Read the model definition and answer for the solid it produces. Units are mm, in the model's axes. Face numbers are marked on the shaded views. A direction names the side the tool comes from. Coordinates: 2 decimals unless noted, no trailing zeros. Order: outer loops, then holes, each group sorted by start corner. A loop starts at its lowest first (then second) coordinate and runs counter-clockwise, first axis right, second up. Notation, with made-up numbers: (29.5, 19.25) -> (77.5, 19.25) arc R30 ccw to (77.5, 45.25) -> close; hole circle Ø4 at (86.5, 56). An arc over 180 degrees is marked (long way). Answer as a JSON object with one key per item and string values. Group by question number.
1) A tool of negligible diameter and unlimited length cuts with its end or side. For the marked faces 1 and 2, from which of +Z, -Z, +X, -X, +Y, -Y can it reach the whole face along a straight path? Write none if from no direction.
2) Section B-B on z = 7 is taken. Determine the outline of the cut face in (x, y), and give its area (3 significant figures).
3) Section D-D on z = 38.5 is taken. Determine the outline of the cut face in (x, y), and give its area (3 significant figures).
4) Section C-C on x = 54 is taken. Determine the outline of the cut face in (y, z) (3 decimals), and give its area (3 significant figures).
5) Section A-A on x = 47.5 is taken. Determine the outline of the cut face in (y, z), and give its area (3 significant figures).
6) Given pin 1 (20 mm diameter, centred on x = 44.5, z = 23.5, fed in from -Y); pin 2 (5 mm diameter, centred on x = 27.5, z = 54.5, fed in from +Y); pin 3 (0.5 mm diameter, centred on x = 55, z = 40.5, fed in from -Y), each flat-ended and moving along its own axis, determine where each tip first touches the part or whether it passes through.
7) Consider L1, parallel to Y at x = 59.5, z = 20 (3 decimals); L2, parallel to Y at x = 18, z = 53.5; L3, parallel to X at y = -6.25, z = 30.5. Determine where each line is inside the solid, lowest interval first.
from build123d import *

# Parameters (mm, degrees)
ESBO_O1_W                                      = 130
ESBO_O1_H                                      = 20
RESSALTO_EXTRUS_O1_DEPTH                       = 95
CORTE_EXTRUS_O2_REACH                          = 22
CORTE_EXTRUS_O3_DEPTH                          = 1
CORTE_EXTRUS_O3_DEPTH_BACK                     = 61
BROCA_DE_ROSQUEAR_DE_CANO_PARA_TARRAXA_D_D     = 6.579997
BROCA_DE_ROSQUEAR_DE_CANO_PARA_TARRAXA_D_DEPTH = 10
BROCA_DE_ROSQUEAR_DE_CANO_PARA_TARRAXA_D_TIP   = 1.976830535
BROCA_DE_ROSQUEAR_DE_CANO_PARA_TARRA_2_D       = 6.579997
BROCA_DE_ROSQUEAR_DE_CANO_PARA_TARRA_2_DEPTH   = 10
BROCA_DE_ROSQUEAR_DE_CANO_PARA_TARRA_2_TIP     = 1.976830535
FILETE2_R                                      = 5
CORTE_EXTRUS_O4_REACH                          = 62
RESSALTO_EXTRUS_O2_REACH                       = 57
ESBO_O13_W                                     = 28
ESBO_O13_H                                     = 8
ESBO_O14_W                                     = 50
ESBO_O14_H                                     = 2
CORTE_EXTRUS_O5_DEPTH                          = 40.5


with BuildPart() as part:
    # Esboço1 → Ressalto-extrusão1 (new body)
    with BuildSketch(Plane.XY):
        Rectangle(ESBO_O1_W, ESBO_O1_H)
    extrude(amount=RESSALTO_EXTRUS_O1_DEPTH)

    # Esboço2 → Corte-extrusão2 (cut, up to next)
    with BuildSketch(Plane(origin=(0, 10, 0), x_dir=(1, 0, 0), z_dir=(0, 1, 0)), mode=Mode.PRIVATE) as corte_extrus_o2_sk1:
        Polygon((15, 0), (-65, 0), (-65, -95), (5, -95), (5, -41), (35, -41), (35, -40), align=None)
    corte_extrus_o2_tool1 = extrude(corte_extrus_o2_sk1.sketch, amount=-CORTE_EXTRUS_O2_REACH, mode=Mode.PRIVATE) & part.part
    add(corte_extrus_o2_tool1.solids().sort_by_distance((-24.897504, 10, 44.887255))[0], mode=Mode.SUBTRACT)

    # Esboço3 → Corte-extrusão3 (cut, two sides)
    with BuildSketch(Plane(origin=(65, 0, 0), x_dir=(0, 0, -1), z_dir=(1, 0, 0))) as corte_extrus_o3_sk:
        Polygon((200.200134404, 50.040026881), (0, 10), (-95, -9), (-295.200134404, -49.040026881), (-375.280188165, 351.360241926), (120.120080642, 450.440295688), align=None)
    extrude(amount=CORTE_EXTRUS_O3_DEPTH, mode=Mode.SUBTRACT)
    extrude(corte_extrus_o3_sk.sketch, amount=-CORTE_EXTRUS_O3_DEPTH_BACK, mode=Mode.SUBTRACT)

    # Broca de rosquear de cano para tarraxa d
    with Locations(Plane(origin=(65, 0, 0), x_dir=(0, 0, -1), z_dir=(1, 0, 0))):
        with Locations((-20, -1.945)):
            Hole(BROCA_DE_ROSQUEAR_DE_CANO_PARA_TARRAXA_D_D / 2, depth=BROCA_DE_ROSQUEAR_DE_CANO_PARA_TARRAXA_D_DEPTH)
            with Locations((0, 0, -(BROCA_DE_ROSQUEAR_DE_CANO_PARA_TARRAXA_D_DEPTH + BROCA_DE_ROSQUEAR_DE_CANO_PARA_TARRAXA_D_TIP / 2))):  # 118° drill point
                Cone(0, BROCA_DE_ROSQUEAR_DE_CANO_PARA_TARRAXA_D_D / 2, BROCA_DE_ROSQUEAR_DE_CANO_PARA_TARRAXA_D_TIP, mode=Mode.SUBTRACT)

    # Broca de rosquear de cano para tarra 2
    with Locations(Plane(origin=(12, 0, -6), x_dir=(0.447213595, 0, 0.894427191), z_dir=(-0.894427191, 0, 0.447213595))):
        with Locations((26.708203932, -1.945)):
            Hole(BROCA_DE_ROSQUEAR_DE_CANO_PARA_TARRA_2_D / 2, depth=BROCA_DE_ROSQUEAR_DE_CANO_PARA_TARRA_2_DEPTH)
            with Locations((0, 0, -(BROCA_DE_ROSQUEAR_DE_CANO_PARA_TARRA_2_DEPTH + BROCA_DE_ROSQUEAR_DE_CANO_PARA_TARRA_2_TIP / 2))):  # 118° drill point
                Cone(0, BROCA_DE_ROSQUEAR_DE_CANO_PARA_TARRA_2_D / 2, BROCA_DE_ROSQUEAR_DE_CANO_PARA_TARRA_2_TIP, mode=Mode.SUBTRACT)

    # Filete2
    filete2_edges = [part.edges().sort_by_distance(p)[0] for p in [
        (65, -9.5, 95),
    ]]
    fillet(filete2_edges, radius=FILETE2_R)

    # Esboço12 → Corte-extrusão4 (cut, up to next)
    with BuildSketch(Plane(origin=(65, 0, 0), x_dir=(0, 0, -1), z_dir=(1, 0, 0)), mode=Mode.PRIVATE) as corte_extrus_o4_sk1:
        Polygon((-41, -10), (-41, 1.8), (-40, 2), (-40, -10), align=None)
    corte_extrus_o4_tool1 = extrude(corte_extrus_o4_sk1.sketch, amount=-CORTE_EXTRUS_O4_REACH, mode=Mode.PRIVATE) & part.part
    add(corte_extrus_o4_tool1.solids().sort_by_distance((65, -4.04986, 40.498599))[0], mode=Mode.SUBTRACT)

    # Esboço13 → Ressalto-extrusão2 (add, up to next)
    with BuildSketch(Plane.XY.offset(40), mode=Mode.PRIVATE) as ressalto_extrus_o2_sk1:
        with Locations((50, -3)):
            Rectangle(ESBO_O13_W, ESBO_O13_H)
    ressalto_extrus_o2_tool1 = extrude(ressalto_extrus_o2_sk1.sketch, amount=RESSALTO_EXTRUS_O2_REACH, mode=Mode.PRIVATE) - part.part
    add(ressalto_extrus_o2_tool1.solids().sort_by_distance((50, -3, 40))[0])

    # Esboço14 → Corte-extrusão5 (cut)
    with BuildSketch(Plane(origin=(0, 0, 0), x_dir=(-1, 0, 0), z_dir=(0, 0, -1))):
        with Locations((-40, -9)):
            Rectangle(ESBO_O14_W, ESBO_O14_H)
    extrude(amount=-CORTE_EXTRUS_O5_DEPTH, mode=Mode.SUBTRACT)


solid = part.part
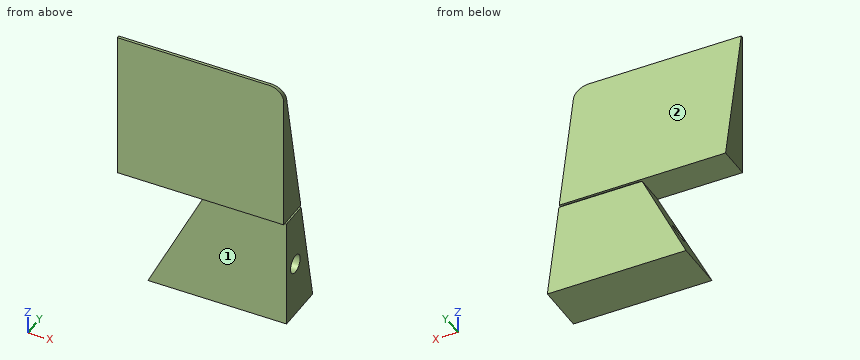
Worked answers:
{
 "1": {"face 1": "-Z, +X, -X, -Y", "face 2": "+Z, +X, -X, +Y"},
 "2": {"outline": "(18.5, -8) -> (65, -8) -> (65, 8.6) -> (18.5, 8.6) -> close", "area": "772 mm²"},
 "3": {"outline": "(34.25, -8) -> (65, -8) -> (65, 2.3) -> (34.25, 2.3) -> close", "area": "317 mm²"},
 "4": {"outline": "(-10, 41) -> (-7, 41) -> (-7, 40) -> (-8, 40) -> (-8, 0) -> (10, 0) -> (2, 40) -> (1, 40) -> (1, 41) -> (1.8, 41) -> (-9, 95) -> (-10, 95) -> close; hole circle Ø3.251 at (-1.945, 20)", "area": "905 mm²"},
 "5": {"outline": "(-10, 41) -> (-7, 41) -> (-7, 40) -> (-8, 40) -> (-8, 0) -> (10, 0) -> (2, 40) -> (1, 40) -> (1, 41) -> (1.8, 41) -> (-9, 95) -> (-10, 95) -> close", "area": "914 mm²"},
 "6": {"pin 1": "stops at y = -8", "pin 2": "stops at y = -0.4", "pin 3": "stops at y = -7"},
 "7": {"L1": "y = -8 to -5.235, 1.345 to 6", "L2": "y = -10 to -0.7", "L3": "x = 30.25 to 65"}
}
